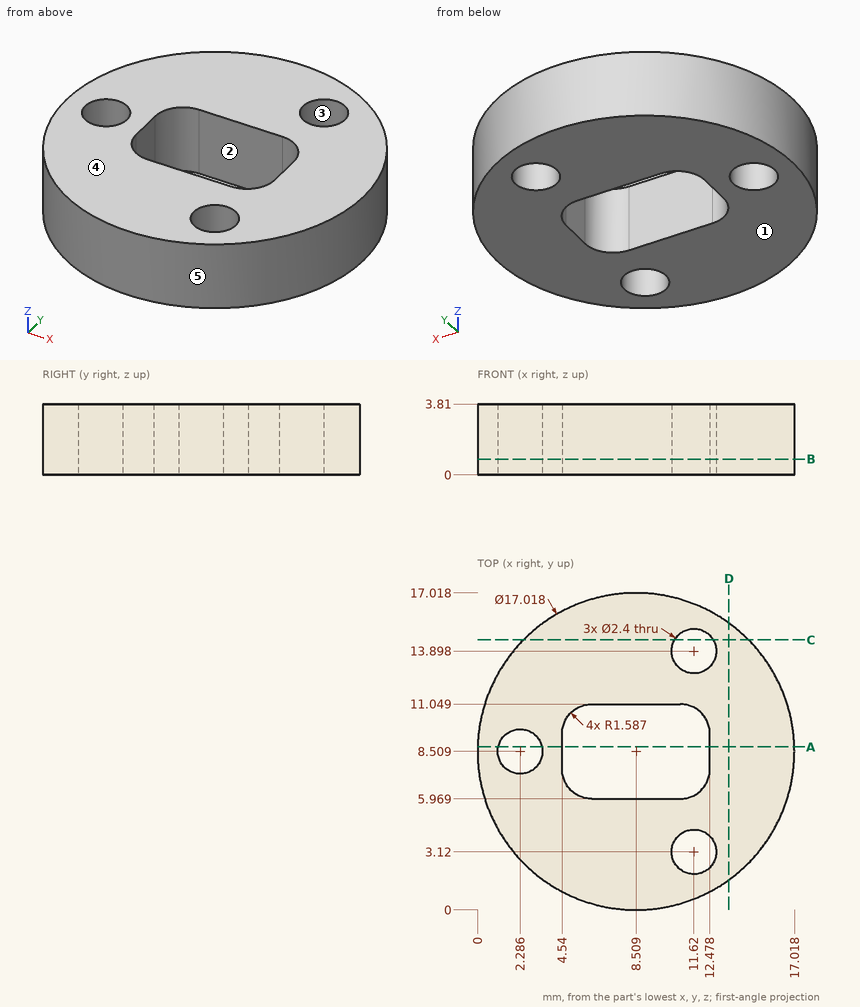
Drawing for the job (mm, zero at the part's lowest x, y, z). A direction names the side the tool comes from. Coordinates: 2 decimals unless noted, no trailing zeros. Order: outer loops, then holes, each group sorted by start corner. A loop starts at its lowest first (then second) coordinate and runs counter-clockwise, first axis right, second up.
Item 1: Band-saw the part on D-D on x = 13.5. List the corners of the cut face in (y, z).
Check sheet entries:
outline: (1.62, 0) - (15.4, 0) - (15.4, 3.81) - (1.62, 3.81) - close
Item 2: Band-saw the part on C-C on y = 14.5. List the corners of the cut face in (x, z).
Check sheet entries:
outline: (2.47, 0) - (10.58, 0) - (10.58, 3.81) - (2.47, 3.81) - close; (12.66, 0) - (14.55, 0) - (14.55, 3.81) - (12.66, 3.81) - close
Item 3: Band-saw the part on A-A on y = 8.75. List the corners of the cut face in (x, z) (1 decimal), plus the area to 3 significant figures.
Check sheet entries:
outline: (0, 0) - (1.1, 0) - (1.1, 3.8) - (0, 3.8) - close; (3.5, 0) - (4.5, 0) - (4.5, 3.8) - (3.5, 3.8) - close; (12.5, 0) - (17, 0) - (17, 3.8) - (12.5, 3.8) - close
area: 25.6 mm2
Item 4: Drill centre lines: L1, parallel to X at y = 9, z = 1.5 (1 decimal); L2, parallel to Y at x = 11.5, z = 2.35 (1 decimal); L3, parallel to X at y = 7.5, z = 2.2 (1 decimal). Where is each one in solid material? Low to high.
Check sheet entries:
L1: x = 0 to 1.2, 3.4 to 4.5, 12.5 to 17
L2: y = 0.5 to 1.9, 4.3 to 6.1, 10.9 to 12.7, 15.1 to 16.5
L3: x = 0.1 to 1.6, 2.9 to 4.5, 12.5 to 17
Item 5: 3-axis set-ups, long thin cutter, end or side, ignore diameter. For the marked faces 1 and 2: which of +Z, -Z, +X, -X, +Y, -Y reach the whole face in a straight line?
Check sheet entries:
face 1: -Z, +X, -X, +Y, -Y
face 2: +Z, -Z
Item 6: Two-plate mould, pull along X, no slides. Class the marked faces 3, 4 and 5: +X half, -X half, draft (parallel to the pull), parting line (faces both ways), or undercut.
Check sheet entries:
face 3: undercut
face 4: draft
face 5: parting line
Item 7: Pin check, flat tips, straight feed: pin 1 Ø0.6 at (y, z) = (8, 1) entering from +X (1 decimal); pin 2 Ø1.5 at (y, z) = (14, 3) entering from -X; pin 3 Ø0.6 at (y, z) = (8, 2.5) entering from -X. Stop position of each tip, or through.
Check sheet entries:
pin 1: stops at x = 17
pin 2: stops at x = 1.44
pin 3: stops at x = 0
Item 8: Band-saw the part on B-B on z = 0.85. Give the number of separate pieces and of enclosed holes in the cut face, plus the area to 3 significant figures.
Check sheet entries:
separate pieces: 1
enclosed holes: 4
area: 176 mm2
